Autodesk Inventor part; units mm, degrees
ref_plane "YZ Plane" through (0, 0, 0) normal (1, 0, 0) x (0, 1, 0)
ref_plane "XZ Plane" through (0, 0, 0) normal (0, 1, 0) x (-1, 0, 0)
ref_plane "XY Plane" through (0, 0, 0) normal (0, 0, 1) x (1, 0, 0)
sketch "Sketch1" plane through (0, 0, 0) normal (0, 1, 0) x (-1, 0, 0)
  line L0 (0, 0) -> (0, -28) construction
  line L1 (-1.5, 0) -> (-1.5, -28)
  line L2 (1.5, -28) -> (1.5, 0)
  arc A0 (1.5, 0) -> (-1.5, 0) centre (0, 0) ccw
  arc A1 (-1.5, -28) -> (1.5, -28) centre (0, -28) ccw
  line L3 (-6.5, 7) -> (12.5, 7)
  line L4 (12.5, 7) -> (12.5, -35)
  line L5 (12.5, -35) -> (-6.5, -35)
  line L6 (-6.5, -35) -> (-6.5, 7)
  line L7 (8.5, 7) -> (8.5, -35)
  circle A2 centre (8.5, -4) radius 1.5
  circle A3 centre (8.5, -24) radius 1.5
  line L8 (0, 1.5) -> (0, -29.5) construction
  line L9 (-3.5, 1.5) -> (-3.5, -29.5)
  line L10 (3.5, -29.5) -> (3.5, 1.5)
  arc A4 (3.5, 1.5) -> (-3.5, 1.5) centre (0, 1.5) ccw
  arc A5 (-3.5, -29.5) -> (3.5, -29.5) centre (0, -29.5) ccw
  circle A6 centre (8.5, 1) radius 1.5
  circle A7 centre (8.5, -29) radius 1.5
  point P0 (0, -14)
  point P1 (0, -14)
  dimension "d0" = 28
  dimension "d1" = 3
  dimension "d2" = 5
  dimension "d3" = 21
  dimension "d4" = 21
  dimension "d5" = 11
  dimension "d6" = 4
  dimension "d7" = 10
  dimension "d8" = 10
  dimension "d9" = 3
  dimension "d10" = 3
  dimension "d11" = 3.5
  dimension "d16" = 5
  dimension "d17" = 5
  dimension "d18" = 3
  dimension "d19" = 3
extrude "Extrusion1" add sketch "Sketch1" along normal blind 5.5 contours L3 L7 A6 A2 A3 A7 L5 L6 | L3 L4 L5 L7 A7 A3 A2 A6 | A4 L10 A5 L9
extrude "Extrusion2" cut sketch "Sketch1" along normal blind 3.5 contours A4 L10 A5 L9
fillet "Fillet1" radius 4 4 edges at (-12.5, 2.75, 7) (-12.5, 2.75, -35) (6.5, 2.75, 7) (6.5, 2.75, -35)
sketch "Sketch2" plane through (0, 5.5, 0) normal (0, 1, 0) x (1, 0, 0)
  arc A0 (6.5, 31) -> (2.5, 35) centre (2.5, 31) ccw
  line L0 (2.5, 35) -> (-8.5, 35)
  arc A1 (-8.5, 35) -> (-12.5, 31) centre (-8.5, 31) ccw
  line L1 (-12.5, 31) -> (-12.5, -3)
  arc A2 (-12.5, -3) -> (-8.5, -7) centre (-8.5, -3) ccw
  line L2 (-8.5, -7) -> (2.5, -7)
  arc A3 (2.5, -7) -> (6.5, -3) centre (2.5, -3) ccw
  line L3 (6.5, -3) -> (6.5, 31)
  circle A4 centre (-8.5, -1) radius 1.5
  circle A5 centre (-8.5, 4) radius 1.5
  circle A6 centre (-8.5, 24) radius 1.5
  circle A7 centre (-8.5, 29) radius 1.5
  arc A8 (-1.5, 0) -> (1.5, 0) centre (0, 0) ccw
  line L4 (-1.5, 0) -> (-1.5, 28)
  arc A9 (1.5, 28) -> (-1.5, 28) centre (0, 28) ccw
  line L5 (1.5, 28) -> (1.5, 0)
  circle A10 centre (-8.5, -1) radius 3.25
  circle A11 centre (-8.5, 4) radius 3.25
  circle A12 centre (-8.5, 24) radius 3.25
  circle A13 centre (-8.5, 29) radius 3.25
  point P0 (-6.4233, 1.5)
  point P1 (-10.5767, 1.5)
  point P2 (-10.5767, 26.5)
  point P3 (-6.4233, 26.5)
  dimension "d21" = 6.5
  dimension "d22" = 6.5
  dimension "d23" = 6.5
  dimension "d24" = 6.5
extrude "Extrusion3" cut sketch "Sketch2" against normal blind 3.5 contours A10 A11 | A11 A10 | A10 A11 | A12 A13 | A13 A12 | A12 A13
properties part number "EStopHolder"
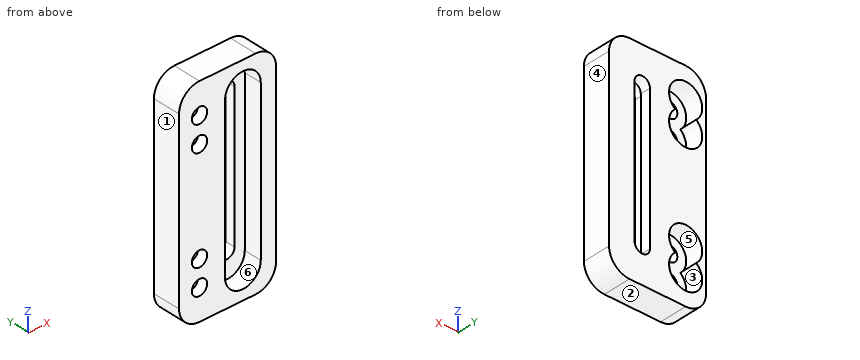
Input: part model. Units: mm. Frame: model coordinates. Face numbers are marked on the shaded views. A direction names the side the tool comes from. Give positions to 0.01 mm unless a question says otherwise; leave off trailing zeros. Loops run counter-clockwise (first coordinate to the right, second up) from the corner with the lowest first, then second, coordinate; pieces in that order, holes last.
1) Mould query, pull axis Z, two halves, no side actions, for the marked faces 1, 2 and 3. Classes: released by +Z, released by -Z, zero draft, split by the parting line, or undercut.
A:
face 1: zero draft
face 2: released by -Z
face 3: undercut
2) Line query: L1, parallel to Z at x = -8.5, y = 0.55; L2, parallel to X at y = 3.7, z = -24; L3, parallel to Z at x = -8.5, y = 4.5. Output: solid intervals per line, ascending.
A:
L1: z = -35 to -30.5, -27.5 to -25.5, -22.5 to -5.5, -2.5 to -0.5, 2.5 to 7
L2: x = -12.5 to -11.75, -5.25 to -1.5, 1.5 to 6.5
L3: z = -35 to -32.25, -20.75 to -7.25, 4.25 to 7
3) Contact query for flat-ended pins moving along their axis: pin 1 (2 mm diameter, centred on x = -10, z = -0.5, fed in from +Y); pin 2 (3.5 mm diameter, centred on x = 0.5, z = -23.5, fed in from -Y). Output: stop coordinate, or through.
A:
pin 1: stops at y = 2
pin 2: stops at y = 3.5
4) Reachability of the marked faces 4, 5 and 6 from +Z, -Z, +X, -X, +Y, -Y: full face, straight path, thin tool, end or side. Return the list, or none.
A:
face 4: +Z, -Z, +X, +Y, -Y
face 5: +Y
face 6: -Y
5) Section query C-C on z = -10.5. Return the cut outline in (x, y).
A:
outline: (-12.5, 0) - (-3.5, 0) - (-3.5, 3.5) - (-1.5, 3.5) - (-1.5, 5.5) - (-12.5, 5.5) - close; (1.5, 3.5) - (3.5, 3.5) - (3.5, 0) - (6.5, 0) - (6.5, 5.5) - (1.5, 5.5) - close
6) Section query A-A on x = 0. Return the cut outline in (y, z), and give its area (3 significant figures).
A:
outline: (0, -35) - (5.5, -35) - (5.5, -29.5) - (3.5, -29.5) - (3.5, -33) - (0, -33) - close; (0, 5) - (3.5, 5) - (3.5, 1.5) - (5.5, 1.5) - (5.5, 7) - (0, 7) - close
area: 36.0 mm2
7) Section query D-D on z = -24. Return the cut outline in (x, y).
A:
outline: (-12.5, 0) - (-10, 0) - (-10, 2) - (-11.75, 2) - (-11.75, 5.5) - (-12.5, 5.5) - close; (-7, 0) - (-3.5, 0) - (-3.5, 3.5) - (-1.5, 3.5) - (-1.5, 5.5) - (-5.25, 5.5) - (-5.25, 2) - (-7, 2) - close; (1.5, 3.5) - (3.5, 3.5) - (3.5, 0) - (6.5, 0) - (6.5, 5.5) - (1.5, 5.5) - close
8) Section query B-B on y = 1.1. Return the cut outline in (x, z), and give its area (3 significant figures).
A:
outline: (-12.5, -31) arc R4 ccw to (-8.5, -35) - (2.5, -35) arc R4 ccw to (6.5, -31) - (6.5, 3) arc R4 ccw to (2.5, 7) - (-8.5, 7) arc R4 ccw to (-12.5, 3) - close; hole circle Ø3 at (-8.5, -29); hole circle Ø3 at (-8.5, -24); hole circle Ø3 at (-8.5, -4); hole circle Ø3 at (-8.5, 1); hole (-3.5, -29.5) arc R3.5 ccw to (3.5, -29.5) - (3.5, 1.5) arc R3.5 ccw to (-3.5, 1.5) - close
area: 501 mm2
